Geometry: final body of the model. Coordinates: model frame, mm. A direction names the side the tool comes from. Give positions to 0.01 mm unless a question says otherwise; leave off trailing zeros. Write each loop counter-clockwise with the first axis right and the second up, starting at its lowest first coordinate (ties: lowest second). Pieces come first, ordered by that corner, then holes.
Q1. Section A-A (x = 10.16). Return the cut outline in (y, z).
Q2. Mould query, pull axis X, two halves, no side actions, for faces 1 (the flat face through (0, 0, 0)), 2 (the flat face through (-2.7, -11, -1)), 3 (the cylindrical face through (-12.1, -13.4, -0.8)), 4 (the flat face through (2.7, -9, -1)). Classes: +X half, -X half, draft (parallel to the pull), parting line (faces both ways), or undercut.
Q3. Reachability of faces 5 (the flat face through (-12.7, 0, -1)), 6 (the flat face through (-2.2, -2, -1)) from +Z, -Z, +X, -X, +Y, -Y: full face, straight path, thin tool, end or side. Return the list, or none.
Q4. Pin query (flat end, axial travel): pin 1 Ø1.8 at (x, y) = (0, -3) entering from -Z. Return the tip coordinate at first contact, or that it passes through.
Q5. Section C-C (z = -0.6). State how many separate pieces and enclosed holes the cut face has, plus the area to 3 significant figures.
Q6. Line query: line 1 (Y direction, x = 2.75, z = -0.3); line 2 (Y direction, x = 2.54, z = -0.3); line 3 (Y direction, x = -2.54, z = -0.45). Output: solid intervals per line, ascending.
Q7. Section B-B (y = 8.89). Return the cut outline in (x, z), plus the area to 3 significant figures.
Autodesk Inventor part; units mm, degrees
ref_plane "YZ Plane" through (0, 0, 0) normal (1, 0, 0) x (0, 1, 0)
ref_plane "XZ Plane" through (0, 0, 0) normal (0, 1, 0) x (-1, 0, 0)
ref_plane "XY Plane" through (0, 0, 0) normal (0, 0, 1) x (1, 0, 0)
ref_plane "作業平面1" through (0, 0, 0) normal (0, 0, 1) x (1, 0, 0)
sketch "スケッチ1" plane through (0, 0, 0) normal (0, 0, 1) x (1, 0, 0)
  line L0 (-12.7, 11.83) -> (-12.7, 13.57)
  line L1 (-12.3, 13.97) -> (-10.56, 13.97)
  line L2 (12.3, -13.97) -> (10.56, -13.97)
  line L3 (12.7, -11.83) -> (12.7, -13.57)
  line L4 (-12.7, 13.97) -> (12.7, 13.97)
  line L5 (12.7, 13.97) -> (12.7, -13.97)
  line L6 (12.7, -13.97) -> (-12.7, -13.97)
  line L7 (-12.7, -13.97) -> (-12.7, 13.97)
  point P0 (0, 0)
extrude "押し出し1" add sketch "スケッチ1" against normal blind 1.6
sketch "スケッチ2" plane through (0, 0, 0) normal (0, 0, 1) x (1, 0, 0)
  circle A0 centre (-10.16, 8.89) radius 1.1
  circle A1 centre (10.16, -3.81) radius 1.1
  point P0 (0, 0)
  dimension "d2" = 2.2
  dimension "d3" = 2.2
  dimension "d4" = 10.16
  dimension "d5" = 8.89
  dimension "d6" = 3.81
  dimension "d7" = 10.16
extrude "押し出し2" cut sketch "スケッチ2" along normal mid plane 20
sketch "スケッチ3" plane through (0, 0, 0) normal (0, 0, 1) x (1, 0, 0)
  circle A0 centre (-2.54, 3.81) radius 0.4
  circle A1 centre (-2.54, 1.27) radius 0.4
  circle A2 centre (2.54, 3.81) radius 0.4
  circle A3 centre (2.54, 1.27) radius 0.4
  point P0 (0, 0)
extrude "押し出し3" cut sketch "スケッチ3" along normal mid plane 20
sketch "スケッチ4" plane through (0, 0, 0) normal (0, 0, 1) x (1, 0, 0)
  circle A0 centre (-2.54, 1.27) radius 0.4
  circle A1 centre (-2.54, 3.81) radius 0.4
  circle A2 centre (2.54, 1.27) radius 0.4
  circle A3 centre (2.54, 3.81) radius 0.4
  circle A4 centre (0, 2.54) radius 0.05
  line L0 (0, -30.1689) -> (0, 24.3248)
  point P0 (0, 0)
  dimension "d12" = 0.1
  dimension "d13" = 2.54
extrude "押し出し4" cut sketch "スケッチ4" against normal blind 20 contours A4 L0 | L0 A4
sketch "スケッチ5" plane through (0, 0, 0) normal (0, 0, 1) x (1, 0, 0)
  circle A0 centre (0, -3) radius 0.8
  circle A1 centre (0, -10) radius 0.8
  point P0 (0, 0)
  dimension "d16" = 1.6
  dimension "d17" = 1.6
  dimension "d18" = 3
  dimension "d19" = 7
extrude "押し出し5" cut sketch "スケッチ5" against normal blind 20
sketch "スケッチ6" plane through (0, 0, 0) normal (0, 0, 1) x (1, 0, 0)
  line L0 (-2.55, -1.3) -> (-2.35, -1.3)
  line L1 (-2.55, -1.3) -> (-2.55, -1.8)
  line L2 (-2.35, -1.8) -> (-2.55, -1.8)
  line L3 (-2.35, -1.8) -> (-2.35, -1.3)
  line L4 (2.55, -8.6) -> (2.55, -9.6)
  line L5 (2.35, -9.6) -> (2.35, -8.6)
  line L6 (-2.35, -10.4) -> (-2.35, -11.4)
  circle A0 centre (0, -3) radius 0.8
  circle A1 centre (0, -10) radius 0.8
  circle A2 centre (0, 2.54) radius 0.05
  circle A3 centre (2.54, 3.81) radius 0.4
  circle A4 centre (-2.54, 3.81) radius 0.4
  circle A5 centre (-2.54, 1.27) radius 0.4
  circle A6 centre (2.54, 1.27) radius 0.4
  circle A7 centre (-10.16, 8.89) radius 1.1
  circle A8 centre (10.16, -3.81) radius 1.1
  line L7 (-12.7, 13.97) -> (12.7, 13.97)
  line L8 (-12.7, -13.97) -> (-12.7, 13.97)
  line L9 (12.7, -13.97) -> (-12.7, -13.97)
  line L10 (12.7, 13.97) -> (12.7, -13.97)
  line L11 (-2.55, -11.4) -> (-2.55, -10.4)
  line L12 (-2.35, -1.8) -> (-2.35, -2.3)
  line L13 (-2.55, -2.3) -> (-2.55, -1.8)
  line L14 (-2.35, -0.8) -> (-2.35, -1.3)
  line L15 (-2.55, -1.3) -> (-2.55, -0.8)
  line L16 (-2.55, -1.3) -> (-2.35, -1.8)
  line L17 (2.35, -8.6) -> (2.55, -9.6)
  line L18 (-2.55, -10.4) -> (-2.35, -11.4)
  line L19 (-2.55, -0.8) -> (-2.35, -0.8)
  line L20 (-2.55, -2.3) -> (-2.35, -2.3)
  line L21 (2.35, -8.6) -> (2.55, -8.6)
  line L22 (2.55, -9.6) -> (2.35, -9.6)
  line L23 (-2.55, -10.4) -> (-2.35, -10.4)
  line L24 (-2.55, -11.4) -> (-2.35, -11.4)
  line L25 (-2.45, -2.3) -> (-2.45, -0.8) construction
  line L26 (-2.2, -2.3) -> (-2.2, -0.8)
  line L27 (-2.7, -0.8) -> (-2.7, -2.3)
  arc A9 (-2.7, -2.3) -> (-2.2, -2.3) centre (-2.45, -2.3) ccw
  arc A10 (-2.2, -0.8) -> (-2.7, -0.8) centre (-2.45, -0.8) ccw
  line L28 (2.45, -9.6) -> (2.45, -8.6) construction
  line L29 (2.7, -9.6) -> (2.7, -8.6)
  line L30 (2.2, -8.6) -> (2.2, -9.6)
  arc A11 (2.2, -9.6) -> (2.7, -9.6) centre (2.45, -9.6) ccw
  arc A12 (2.7, -8.6) -> (2.2, -8.6) centre (2.45, -8.6) ccw
  line L31 (-2.45, -11.4) -> (-2.45, -10.4) construction
  line L32 (-2.2, -11.4) -> (-2.2, -10.4)
  line L33 (-2.7, -10.4) -> (-2.7, -11.4)
  arc A13 (-2.7, -11.4) -> (-2.2, -11.4) centre (-2.45, -11.4) ccw
  arc A14 (-2.2, -10.4) -> (-2.7, -10.4) centre (-2.45, -10.4) ccw
  point P0 (0, 0)
  point P1 (-2.45, -1.55)
  point P2 (2.45, -9.1)
  point P3 (-2.45, -10.9)
  dimension "d22" = 0.2
  dimension "d23" = 0.5
  dimension "d24" = 0.5
  dimension "d25" = 0.5
extrude "押し出し6" cut sketch "スケッチ6" against normal blind 2 contours L15 L19 L14 L0 | L16 L2 L1 | L0 L3 L16 | L2 L12 L20 L13 | L4 L17 L21 | L22 L5 L17 | L6 L18 L23 | L24 L11 L18 | A9 L27 A10 L26 | A11 L30 A12 L29 | A13 L33 A14 L32
fillet "フィレット1" radius 2 4 edges at (-12.7, -13.97, -0.8) (12.7, -13.97, -0.8) (12.7, 13.97, -0.8) (-12.7, 13.97, -0.8)
move faces "移動1" translate (0, 0.52, 0) faces at (-2.1452, 1.2058, -0.5333) (2.9348, 1.2058, -0.5333)
move faces "移動2" translate (0, -0.52, 0) faces at (-2.1452, 3.7458, -0.5333) (2.9348, 3.7458, -0.5333)
properties part number "HbSensorBoard01"
Computed:
1. outline: (-13.97, -1.6) - (-4.91, -1.6) - (-4.91, 0) - (-13.97, 0) - close; (-2.71, -1.6) - (13.97, -1.6) - (13.97, 0) - (-2.71, 0) - close
2. face 1: draft
2. face 2: undercut
2. face 3: -X half
2. face 4: undercut
3. face 5: +Z, -Z, -X, +Y, -Y
3. face 6: +Z, -Z
4. pin 1: stops at z = -1.6
5. separate pieces: 1
5. enclosed holes: 12
5. area: 690 mm2
6. line 1: y = -13.97 to 1.45, 2.13 to 2.95, 3.63 to 13.97
6. line 2: y = -13.97 to -9.83, -8.37 to 1.39, 2.19 to 2.89, 3.69 to 13.97
6. line 3: y = -13.97 to -11.63, -10.17 to -2.53, -0.57 to 1.39, 2.19 to 2.89, 3.69 to 13.97
7. outline: (-12.7, -1.6) - (-11.26, -1.6) - (-11.26, 0) - (-12.7, 0) - close; (-9.06, -1.6) - (12.7, -1.6) - (12.7, 0) - (-9.06, 0) - close
7. area: 37.1 mm2
